The model under review builds one solid part; all positions refer to its coordinate system, in mm. Face numbers are marked on the shaded views. A direction names the side the tool comes from. Coordinates: 2 decimals unless noted, no trailing zeros. Loops run counter-clockwise (first coordinate to the right, second up) from the corner with the lowest first, then second, coordinate; pieces in that order, holes last. Notation, with made-up numbers: (10.5, -37) - (28.5, -37) arc R13 ccw to (28.5, -22) - close; hole circle Ø7 at (55.5, 7). An arc over 180 degrees is marked (long way). One line per item, written item: value. Start each with the question number.
1. Insertion check: P1, Ø3, axis at x = 0, z = 0, coming from the +Y side; P2, Ø1.4, axis at x = -0.5, z = 0, coming from the -Y side; P3, Ø6, axis at x = -2.5, y = 8.5, coming from the -Z side. Each pin has a flat end and moves straight along its axis. Give the tip position at first contact, or say it passes through.
2. We need section C-C, the plane x = 0. Give the boundary of the cut face in (y, z) (3 decimals), then the cut area to 3 significant figures.
3. We need section A-A, the plane z = 0. Give the boundary of the cut face in (x, y) (3 decimals).
4. We need section B-B, the plane y = 27. Give the boundary of the cut face in (x, z).
5. To check wall thickness, follow line 1 (X direction, y = 3.25, z = 0) (3 decimals); line 2 (X direction, y = 67.9, z = 0); line 3 (Y direction, x = -1.5, z = 3). State the ranges of each line that lie inside material, in increasing order.
6. For the marked faces 1 and 2, list the 3-axis set-ups (+Z, -Z, +X, -X, +Y, -Y) from which the entire face can be reached by the end or side of a thin tool; tool diameter is ignored.
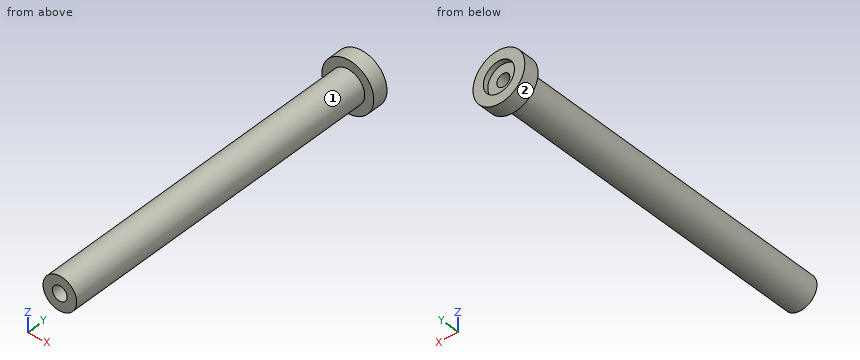
from build123d import *

# Parameters (mm, degrees)
SKETCH1_R           = 3.25
BOSS_EXTRUDE1_DEPTH = 65.3
SKETCH2_R           = 5
BOSS_EXTRUDE2_DEPTH = 3
SKETCH3_R           = 1.425
CUT_EXTRUDE1_DEPTH  = 9
SHELL1_T            = -2


with BuildPart() as part:
    # Sketch1 → Boss-Extrude1 (new body)
    with BuildSketch(Plane(origin=(0, 0, 0), x_dir=(1, 0, 0), z_dir=(0, 1, 0))):
        with Locations(Location((0, 0, 0), (0, 0, 270))):
            Circle(SKETCH1_R)
    extrude(amount=BOSS_EXTRUDE1_DEPTH)

    # Sketch2 → Boss-Extrude2 (add)
    with BuildSketch(Plane(origin=(0, 65.3, 0), x_dir=(1, 0, 0), z_dir=(0, 1, 0))):
        with Locations(Location((0, 0, 0), (0, 0, 270))):
            Circle(SKETCH2_R)
    extrude(amount=BOSS_EXTRUDE2_DEPTH)

    # Sketch3 → Cut-Extrude1 (cut)
    with BuildSketch(Plane.XZ):
        with Locations(Location((0, 0, 0), (0, 0, 270))):
            Circle(SKETCH3_R)
    extrude(amount=-CUT_EXTRUDE1_DEPTH, mode=Mode.SUBTRACT)

    # Shell1
    shell1_openings = [part.faces().sort_by_distance(p)[0] for p in [
        (0, 68.3, 0),
    ]]
    offset(amount=SHELL1_T, openings=shell1_openings, kind=Kind.INTERSECTION)


solid = part.part
Findings below:
1. P1: y = 67.3
1. P2: y = 9
1. P3: z = -3.25
2. outline: (0, -3.25) - (65.3, -3.25) - (65.3, -5) - (68.3, -5) - (68.3, -3) - (67.3, -3) - (67.3, -1.25) - (11, -1.25) - (11, 1.25) - (67.3, 1.25) - (67.3, 3) - (68.3, 3) - (68.3, 5) - (65.3, 5) - (65.3, 3.25) - (0, 3.25) - (0, 1.425) - (9, 1.425) - (9, -1.425) - (0, -1.425) - close
2. area: 282 mm2
3. outline: (-5, 65.3) - (-3.25, 65.3) - (-3.25, 0) - (-1.425, 0) - (-1.425, 9) - (1.425, 9) - (1.425, 0) - (3.25, 0) - (3.25, 65.3) - (5, 65.3) - (5, 68.3) - (3, 68.3) - (3, 67.3) - (1.25, 67.3) - (1.25, 11) - (-1.25, 11) - (-1.25, 67.3) - (-3, 67.3) - (-3, 68.3) - (-5, 68.3) - close
4. outline: circle Ø6.5 at (0, 0); hole circle Ø2.5 at (0, 0)
5. line 1: -3.25 to -1.425, 1.425 to 3.25
5. line 2: -5 to -3, 3 to 5
5. line 3: 65.3 to 68.3
6. face 1: -Y
6. face 2: +Y, -Y
